Can you work these out from the model? Positions are in its coordinate system, mm. A direction names the side the tool comes from. Round coordinates to 2 decimals unless told otherwise and drop trailing zeros. Write each loop counter-clockwise with the first axis right and the second up, starting at its lowest first coordinate (ties: lowest second). Pieces come first, ordered by that corner, then holes. Notation, with made-up numbers: (18, -8) -> (50, -8) arc R32 ccw to (50, 27) -> close; hole circle Ø11 at (68, 73). An arc over 180 degrees is marked (long way). Write item = value, one per line. Start each with the question number.
1) Imagine slicing it at A-A, the plane x = -23.5. Please give me the cut outline in (y, z), then the cut area to 3 significant figures.
2) I'm going to push flat-ended pins straight in: pin 1 (1.2 mm diameter, centred on x = -44.5, z = 2.5, fed in from +Y); pin 2 (2 mm diameter, centred on y = 4, z = 1.5, fed in from -X); pin 3 (1 mm diameter, centred on x = 13.5, z = 0.5, fed in from +Y). Where does each tip first touch, or does it pass through?
3) Imagine slicing it at B-B, the plane x = -0.5. State how many separate pieces and enclosed holes the cut face has, then the cut area to 3 significant figures.
4) If I drill on line 1 (Y direction, x = 0, z = 2.25); line 2 (Y direction, x = 2.5, z = 1.85); line 3 (Y direction, x = -31.5, z = 2.1), over which ranges is the centre line in solid material (lowest first)?
5) For faces 1 (the face through (11, 1, 0)), 2 (the face through (-31.14, -25.87, 2.03)), which set-ups out of +Z, -Z, +X, -X, +Y, -Y let a thin tool reach every point of the face, with its end or its side?
6) Thinking about a two-plate mould opening in Y: for faces 3 (the face through (38.11, -13.66, 2.03)), 4 (the face through (-6.837, -39.904, 2.028)), 5 (the face through (8.637, -49.248, 1.972)), 6 (the face through (-46.97, 17.14, 1.97)), which applies, +Y half, -Y half, draft (parallel to the pull), parting line (faces both ways), or undercut?
from build123d import *

# Parameters (mm, degrees)
SKETCH1_R           = 50
BOSS_EXTRUDE1_DEPTH = 4
SKETCH2_W           = 6.3
SKETCH2_H           = 28
CUT_EXTRUDE1_DEPTH  = 4
SKETCH5_W           = 0.4
SKETCH5_H           = 28
CUT_EXTRUDE2_DEPTH  = 1.8
SKETCH7_W           = 0.4
SKETCH7_H           = 28
CUT_EXTRUDE3_DEPTH  = 1.8
SKETCH8_W           = 0.5
SKETCH8_H           = 28
SKETCH9_W           = 0.5
SKETCH9_H           = 28
SKETCH10_W          = 28
SKETCH10_H          = 0.5
SKETCH11_W          = 28
SKETCH11_H          = 0.5
SKETCH12_W          = 0.5
SKETCH12_H          = 28
SKETCH13_W          = 0.5
SKETCH13_H          = 28
SKETCH14_W          = 28
SKETCH14_H          = 0.5
SKETCH15_W          = 0.5
SKETCH15_H          = 28
SKETCH16_W          = 28
SKETCH16_H          = 0.5
SKETCH17_R          = 3.2
CUT_EXTRUDE4_DEPTH  = 10


with BuildPart() as part:
    # Sketch1 → Boss-Extrude1 (new body)
    with BuildSketch(Plane.XY):
        Circle(SKETCH1_R)
    extrude(amount=BOSS_EXTRUDE1_DEPTH)

    # Sketch2 → Cut-Extrude1 (cut)
    with BuildSketch(Plane.XY.offset(4)):
        Polygon((5.663242619, 48.504941857), (6.757226139, 42.300653013), (-20.817390946, 37.438504038), (-21.911374465, 43.642792882), align=None)
        with BuildLine():
            Line((5.593783348, 48.898864958), (5.452196014, 49.701846632))
            ThreePointArc((5.452196014, 49.701846632), (-8.682408883, 49.240387651), (-22.12242107, 44.839697657))
            Line((-22.12242107, 44.839697657), (-21.980833736, 44.036715983))
            Line((-21.980833736, 44.036715983), (5.593783348, 48.898864958))
        make_face()
        Polygon((35.516671173, 33.516678987), (32.366671173, 28.060718943), (8.117959867, 42.060718943), (11.267959867, 47.516678987), align=None)
        Polygon((33.254827036, 27.002256002), (42.831391049, 0.69086262), (48.75145456, 2.845589522), (39.174890547, 29.156982905), align=None)
        with BuildLine():
            Line((40.316963791, 29.572663571), (39.550767596, 29.293790962))
            Line((39.550767596, 29.293790962), (49.127331609, 2.98239758))
            Line((49.127331609, 2.98239758), (49.893527804, 3.261270189))
            ThreePointArc((49.893527804, 3.261270189), (46.984631039, 17.101007166), (40.316963791, 29.572663571))
        make_face()
        with BuildLine():
            ThreePointArc((40.316963791, -29.572663571), (46.984631039, -17.101007166), (49.893527804, -3.261270189))
            Line((49.893527804, -3.261270189), (49.127331609, -2.98239758))
            Line((49.127331609, -2.98239758), (39.550767596, -29.293790962))
            Line((39.550767596, -29.293790962), (40.316963791, -29.572663571))
        make_face()
        Polygon((32.366671173, -28.060718943), (8.117959867, -42.060718943), (11.267959867, -47.516678987), (35.516671173, -33.516678987), align=None)
        with BuildLine():
            ThreePointArc((-22.12242107, -44.839697657), (-8.682408883, -49.240387651), (5.452196014, -49.701846632))
            Line((5.452196014, -49.701846632), (5.593783348, -48.898864958))
            Line((5.593783348, -48.898864958), (-21.980833736, -44.036715983))
            Line((-21.980833736, -44.036715983), (-22.12242107, -44.839697657))
        make_face()
        Polygon((6.757226139, -42.300653013), (-20.817390946, -37.438504038), (-21.911374465, -43.642792882), (5.663242619, -48.504941857), align=None)
        with BuildLine():
            Line((-45.144550944, -19.605073996), (-45.769159805, -20.129183061))
            ThreePointArc((-45.769159805, -20.129183061), (-38.302222156, -32.139380484), (-27.771106734, -41.578427469))
            Line((-27.771106734, -41.578427469), (-27.146497873, -41.054318403))
            Line((-27.146497873, -41.054318403), (-45.144550944, -19.605073996))
        make_face()
        Polygon((-44.838133167, -19.347958952), (-40.012053175, -15.298397011), (-22.014000104, -36.747641418), (-26.840080095, -40.797203359), align=None)
        with BuildLine():
            Line((-47.184631039, 14), (-48, 14))
            ThreePointArc((-48, 14), (-50, 0), (-48, -14))
            Line((-48, -14), (-47.184631039, -14))
            Line((-47.184631039, -14), (-47.184631039, 14))
        make_face()
        with Locations((-43.634631039, 0)):
            Rectangle(SKETCH2_W, SKETCH2_H)
        Polygon((-26.840080095, 40.797203359), (-22.014000104, 36.747641418), (-40.012053175, 15.298397011), (-44.838133167, 19.347958952), align=None)
        with BuildLine():
            Line((-27.146497873, 41.054318403), (-27.771106734, 41.578427469))
            ThreePointArc((-27.771106734, 41.578427469), (-38.302222156, 32.139380484), (-45.769159805, 20.129183061))
            Line((-45.769159805, 20.129183061), (-45.144550944, 19.605073996))
            Line((-45.144550944, 19.605073996), (-27.146497873, 41.054318403))
        make_face()
        with BuildLine():
            ThreePointArc((36.124355653, 34.569219382), (25, 43.301270189), (11.875644347, 48.569219382))
            Line((11.875644347, 48.569219382), (11.467959867, 47.863089148))
            Line((11.467959867, 47.863089148), (35.716671173, 33.863089148))
            Line((35.716671173, 33.863089148), (36.124355653, 34.569219382))
        make_face()
        Polygon((42.831391049, -0.69086262), (33.254827036, -27.002256002), (39.174890547, -29.156982905), (48.75145456, -2.845589522), align=None)
        with BuildLine():
            Line((11.467959867, -47.863089148), (35.716671173, -33.863089148))
            Line((35.716671173, -33.863089148), (36.124355653, -34.569219382))
            ThreePointArc((36.124355653, -34.569219382), (25, -43.301270189), (11.875644347, -48.569219382))
            Line((11.875644347, -48.569219382), (11.467959867, -47.863089148))
        make_face()
    extrude(amount=-CUT_EXTRUDE1_DEPTH, mode=Mode.SUBTRACT)

    # Sketch5 → Cut-Extrude2 (cut)
    with BuildSketch(Plane.XY.offset(4)):
        Polygon((39.174890547, 29.156982905), (39.550767596, 29.293790962), (49.127331609, 2.98239758), (48.75145456, 2.845589522), align=None)
        Polygon((39.174890547, -29.156982905), (39.550767596, -29.293790962), (49.127331609, -2.98239758), (48.75145456, -2.845589522), align=None)
        Polygon((11.267959867, -47.516678987), (11.467959867, -47.863089148), (35.716671173, -33.863089148), (35.516671173, -33.516678987), align=None)
        Polygon((-21.911374465, -43.642792882), (-21.980833736, -44.036715983), (5.593783348, -48.898864958), (5.663242619, -48.504941857), align=None)
        Polygon((-27.146497873, -41.054318403), (-26.840080095, -40.797203359), (-44.838133167, -19.347958952), (-45.144550944, -19.605073996), align=None)
        with Locations((-46.984631039, 0)):
            Rectangle(SKETCH5_W, SKETCH5_H)
        Polygon((-45.144550944, 19.605073996), (-44.838133167, 19.347958952), (-26.840080095, 40.797203359), (-27.146497873, 41.054318403), align=None)
        Polygon((-21.980833736, 44.036715983), (-21.911374465, 43.642792882), (5.663242619, 48.504941857), (5.593783348, 48.898864958), align=None)
        Polygon((11.267959867, 47.516678987), (11.467959867, 47.863089148), (35.716671173, 33.863089148), (35.516671173, 33.516678987), align=None)
    extrude(amount=-CUT_EXTRUDE2_DEPTH, mode=Mode.SUBTRACT)

    # Sketch7 → Cut-Extrude3 (cut)
    with BuildSketch(Plane(origin=(0, 0, 0), x_dir=(-1, 0, 0), z_dir=(0, 0, -1))):
        with Locations((46.984631039, 0)):
            Rectangle(SKETCH7_W, SKETCH7_H)
        Polygon((44.838133167, -19.347958952), (45.144550944, -19.605073996), (27.146497873, -41.054318403), (26.840080095, -40.797203359), align=None)
        Polygon((21.911374465, -43.642792882), (21.980833736, -44.036715983), (-5.593783348, -48.898864958), (-5.663242619, -48.504941857), align=None)
        Polygon((-11.267959867, -47.516678987), (-11.467959867, -47.863089148), (-35.716671173, -33.863089148), (-35.516671173, -33.516678987), align=None)
        Polygon((-39.174890547, -29.156982905), (-39.550767596, -29.293790962), (-49.127331609, -2.98239758), (-48.75145456, -2.845589522), align=None)
        Polygon((-48.75145456, 2.845589522), (-49.127331609, 2.98239758), (-39.550767596, 29.293790962), (-39.174890547, 29.156982905), align=None)
        Polygon((-35.716671173, 33.863089148), (-11.467959867, 47.863089148), (-11.267959867, 47.516678987), (-35.516671173, 33.516678987), align=None)
        Polygon((-5.593783348, 48.898864958), (-5.663242619, 48.504941857), (21.911374465, 43.642792882), (21.980833736, 44.036715983), align=None)
        Polygon((27.146497873, 41.054318403), (26.840080095, 40.797203359), (44.838133167, 19.347958952), (45.144550944, 19.605073996), align=None)
    extrude(amount=-CUT_EXTRUDE3_DEPTH, mode=Mode.SUBTRACT)

    # Sketch8 → Revolve1 (revolve)
    with BuildSketch(Plane.ZY.offset(46.984631039)):
        with Locations((2.25, 0)):
            Rectangle(SKETCH8_W, SKETCH8_H)
    revolve(axis=Axis((-46.984631039, 14, 2), (0, -1, 0)))

    # Sketch9 → Revolve2 (revolve)
    with BuildSketch(Plane(origin=(-35.99231552, 30.201138678, 0), x_dir=(0, 0, 1), z_dir=(-0.766044443, 0.64278761, 0))):
        with Locations((2.25, 0)):
            Rectangle(SKETCH9_W, SKETCH9_H)
    revolve(axis=Axis((-26.993288984, 40.925760881, 2), (-0.64278761, -0.766044443, 0)))

    # Sketch10 → Revolve3 (revolve)
    with BuildSketch(Plane(origin=(-8.158795558, 46.27082892, 0), x_dir=(0.984807753, 0.173648178, 0), z_dir=(-0.173648178, 0.984807753, 0))):
        with Locations((0, -1.75)):
            Rectangle(SKETCH10_W, SKETCH10_H)
    revolve(axis=Axis((-21.9461041, 43.839754433, 2), (0.984807753, 0.173648178, 0)))

    # Sketch11 → Revolve4 (revolve)
    with BuildSketch(Plane(origin=(23.49231552, 40.689884067, 0), x_dir=(0.866025404, -0.5, 0), z_dir=(0.5, 0.866025404, 0))):
        with Locations((0, -1.75)):
            Rectangle(SKETCH11_W, SKETCH11_H)
    revolve(axis=Axis((11.367959867, 47.689884067, 2), (0.866025404, -0.5, 0)))

    # Sketch12 → Revolve5 (revolve)
    with BuildSketch(Plane(origin=(44.151111078, 16.069690242, 0), x_dir=(0, 0, -1), z_dir=(0.939692621, 0.342020143, 0))):
        with Locations((-1.75, 0)):
            Rectangle(SKETCH12_W, SKETCH12_H)
    revolve(axis=Axis((39.362829071, 29.225386933, 2), (0.342020143, -0.939692621, 0)))

    # Sketch13 → Revolve6 (revolve)
    with BuildSketch(Plane(origin=(44.151111078, -16.069690242, 0), x_dir=(0, 0, -1), z_dir=(0.939692621, -0.342020143, 0))):
        with Locations((-1.75, 0)):
            Rectangle(SKETCH13_W, SKETCH13_H)
    revolve(axis=Axis((48.939393085, -2.913993551, 2), (-0.342020143, -0.939692621, 0)))

    # Sketch14 → Revolve7 (revolve)
    with BuildSketch(Plane(origin=(23.49231552, -40.689884067, 0), x_dir=(-0.866025404, -0.5, 0), z_dir=(0.5, -0.866025404, 0))):
        with Locations((0, -2.25)):
            Rectangle(SKETCH14_W, SKETCH14_H)
    revolve(axis=Axis((11.367959867, -47.689884067, 2), (0.866025404, 0.5, 0)))

    # Sketch15 → Revolve8 (revolve)
    with BuildSketch(Plane(origin=(-35.99231552, -30.201138678, 0), x_dir=(0, 0, 1), z_dir=(-0.766044443, -0.64278761, 0))):
        with Locations((2.25, 0)):
            Rectangle(SKETCH15_W, SKETCH15_H)
    revolve(axis=Axis((-44.991342055, -19.476516474, 2), (0.64278761, -0.766044443, 0)))

    # Sketch16 → Revolve9 (revolve)
    with BuildSketch(Plane(origin=(-8.158795558, -46.27082892, 0), x_dir=(-0.984807753, 0.173648178, 0), z_dir=(-0.173648178, -0.984807753, 0))):
        with Locations((0, -1.75)):
            Rectangle(SKETCH16_W, SKETCH16_H)
    revolve(axis=Axis((5.628512984, -48.701903407, 2), (-0.984807753, 0.173648178, 0)))

    # Sketch17 → Cut-Extrude4 (cut)
    with BuildSketch(Plane(origin=(0, 0, 0), x_dir=(-1, 0, 0), z_dir=(0, 0, -1))):
        Circle(SKETCH17_R)
    extrude(amount=-CUT_EXTRUDE4_DEPTH, mode=Mode.SUBTRACT)


solid = part.part
Reported:
q1.outline = (-44.13, 0) -> (-37.99, 0) -> (-37.99, 4) -> (-44.13, 4) -> close; (-34.98, 0) -> (34.98, 0) -> (34.98, 4) -> (-34.98, 4) -> close; (37.99, 0) -> (44.13, 0) -> (44.13, 4) -> (37.99, 4) -> close
q1.area = 329 mm²
q2.pin_1 = 21.39
q2.pin_2 = -47.48
q2.pin_3 = 39.24
q3.separate_pieces = 4
q3.enclosed_holes = 0
q3.area = 304 mm²
q4.line_1 = -48.15 to -47.27, -41.11 to -3.2, 3.2 to 41.11, 47.27 to 48.15
q4.line_2 = -48.63 to -47.67, -41.55 to -2, 2 to 41.55, 47.67 to 48.63
q4.line_3 = -36.32 to -34.79, -25.44 to 25.44, 34.79 to 36.32
q5.face_1 = -Z, +X, -X, +Y, -Y
q5.face_2 = +Z, -Z
q6.face_3 = undercut
q6.face_4 = undercut
q6.face_5 = -Y half
q6.face_6 = +Y half
